```python
from build123d import *

# Parameters (mm, degrees)
SKETCH_W            = 110
SKETCH_H            = 110
PAD_DEPTH           = 1.5
PAD001_DEPTH        = 1
SKETCH002_R         = 6
SKETCH002_R_2       = 1.5
SKETCH002_R_3       = 5
SKETCH002_W         = 12
SKETCH002_H         = 7
SKETCH002_W_2       = 10
SKETCH002_H_2       = 1
PAD002_DEPTH        = 1
LINEARPATTERN_COUNT = 4
LINEARPATTERN_PITCH = 26.67


with BuildPart() as part:
    # Sketch → Pad (new body)
    with BuildSketch(Plane.XY):
        Rectangle(SKETCH_W, SKETCH_H)
    extrude(amount=PAD_DEPTH)

    # Sketch001 → Pad001 (join)
    with BuildSketch(Plane(origin=(0, 0, 0), x_dir=(1, 0, 0), z_dir=(0, 0, -1))):
        with BuildLine():
            Line((-49.8, 53.8), (49.8, 53.8))
            ThreePointArc((53.8, 49.8), (52.628427, 52.628427), (49.8, 53.8))
            Line((53.8, 49.8), (53.8, -49.8))
            ThreePointArc((49.8, -53.8), (52.628427, -52.628427), (53.8, -49.8))
            Line((49.8, -53.8), (-49.8, -53.8))
            ThreePointArc((-53.8, -49.8), (-52.628427, -52.628427), (-49.8, -53.8))
            Line((-53.8, -49.8), (-53.8, 49.8))
            ThreePointArc((-49.8, 53.8), (-52.628427, 52.628427), (-53.8, 49.8))
        make_face()
        with BuildLine():
            Line((-49.8, 52.8), (49.8, 52.8))
            ThreePointArc((52.8, 49.8), (51.92132, 51.92132), (49.8, 52.8))
            Line((52.8, 49.8), (52.8, -49.8))
            ThreePointArc((49.8, -52.8), (51.92132, -51.92132), (52.8, -49.8))
            Line((49.8, -52.8), (-49.8, -52.8))
            ThreePointArc((-52.8, -49.8), (-51.92132, -51.92132), (-49.8, -52.8))
            Line((-52.8, -49.8), (-52.8, 49.8))
            ThreePointArc((-49.8, 52.8), (-51.92132, 51.92132), (-52.8, 49.8))
        make_face(mode=Mode.SUBTRACT)
    extrude(amount=PAD001_DEPTH)

    # Sketch002 → Pad002 (join)
    with BuildSketch(Plane(origin=(0, 0, 0), x_dir=(1, 0, 0), z_dir=(0, 0, -1))):
        with Locations((-40.005, 40.005)):
            Circle(SKETCH002_R)
        with BuildLine():
            ThreePointArc((-36.42415, 36.515371), (-43.218938, 43.835222), (-37.190194, 35.872583))
            Line((-37.190194, 35.872583), (-38.925721, 37.940903))
            ThreePointArc((-38.888744, 38.363553), (-38.994766, 38.159886), (-38.925721, 37.940903))
            Line((-38.888744, 38.363553), (-38.582326, 38.620668))
            ThreePointArc((-38.159676, 38.583691), (-38.363343, 38.689713), (-38.582326, 38.620668))
            Line((-36.42415, 36.515371), (-38.159676, 38.583691))
        make_face(mode=Mode.SUBTRACT)
        with Locations((-40.005, 49.505)):
            Circle(SKETCH002_R_2)
        with Locations((-40.005, 25)):
            Circle(SKETCH002_R_2)
        with Locations((-40.005, -30.505)):
            Circle(SKETCH002_R_2)
        with Locations((-40.005, -40.005)):
            Circle(SKETCH002_R_3)
        with BuildLine():
            ThreePointArc((-39.255, 18.1), (-40.005, 18.85), (-40.755, 18.1))
            Line((-40.755, 18.1), (-40.755, 4.5))
            Line((-40.755, 4.5), (-39.255, 4.5))
            Line((-39.255, 18.1), (-39.255, 4.5))
        make_face()
        with BuildLine():
            ThreePointArc((-40.755, -18.1), (-40.005, -18.85), (-39.255, -18.1))
            Line((-39.255, -4.5), (-39.255, -18.1))
            Line((-40.755, -4.5), (-39.255, -4.5))
            Line((-40.755, -18.1), (-40.755, -4.5))
        make_face()
        with Locations((-40.005, 0)):
            Rectangle(SKETCH002_W, SKETCH002_H)
        with Locations((-40.005, 0)):
            Rectangle(SKETCH002_W_2, SKETCH002_H_2, mode=Mode.SUBTRACT)
    pad002 = extrude(amount=PAD002_DEPTH)

    # LinearPattern: Pad002 ×4
    with Locations(*[(i * LINEARPATTERN_PITCH, 0, 0) for i in range(1, LINEARPATTERN_COUNT)]):
        add(pad002)


solid = part.part
```
Geometry check sheet. Reference: the model listing, model coordinates, mm. A direction names the side the tool comes from. Coordinates: 2 decimals unless noted, no trailing zeros. Order: outer loops, then holes, each group sorted by start corner. A loop starts at its lowest first (then second) coordinate and runs counter-clockwise, first axis right, second up. Notation, with made-up numbers: (-33, -5) - (-20, -5) arc R29 ccw to (-20, 24) - close; hole circle Ø9 at (-15, 12). An arc over 180 degrees is marked (long way). Answer in a Markdown table with one row per item. Add a question column.
1. Draft check along Y on faces 3 (the face through (-13, 30, -1)), 4 (the face through (40.697, 31.836, -0.493)). Enter one of: +Y half, -Y half, draft (parallel to the pull), parting line (faces both ways), or undercut.
2. Material ranges on L1, parallel to X at y = -14, z = -0.05 (3 decimals); L2, parallel to Z at x = 14.5, y = 25; L3, parallel to Y at x = -8, z = -0.1, recorded low to high. Write a range as [from, to].
3. Section check A-A (y = 24.5). Enter the section's corners in (x, z), plus the area to 3 significant figures.
4. Access from +Z, -Z, +X, -X, +Y, -Y to the whole of each face (thin tool, end or side, straight path). Record for faces 1 (the face through (-51.94, 51.9, -0.49)), 2 (the face through (-13, -25, -1)).
5. Gauge pin test, flat ends, axial feed: pin 1 Ø0.8 at (y, z) = (-0.5, -0.5) entering from +X; pin 2 Ø0.8 at (x, y) = (-15.5, 0) entering from -Z; pin 3 Ø0.5 at (y, z) = (13, -0.5) entering from -X. Record the tip position at first contact, or that the pin passes through.
6. Section check C-C (y = -25). Enter the section's corners in (x, z) (3 decimals), plus the area to 3 significant figures.
Data:
| question | item | result |
|---|---|---|
| 1 | face 3 | draft |
| 1 | face 4 | undercut |
| 2 | L1 | x = [-53.8, -52.8], [-40.755, -39.255], [-14.085, -12.585], [12.585, 14.085], [39.255, 40.755], [52.8, 53.8] |
| 2 | L2 | z = [0, 1.5] |
| 2 | L3 | y = [-53.8, -52.8], [-42.75, -37.26], [-3.5, 3.5], [52.8, 53.8] |
| 3 | outline | (-55, 0) - (-53.8, 0) - (-53.8, -1) - (-52.8, -1) - (-52.8, 0) - (52.8, 0) - (52.8, -1) - (53.8, -1) - (53.8, 0) - (55, 0) - (55, 1.5) - (-55, 1.5) - close |
| 3 | area | 167 mm² |
| 4 | face 1 | -Z |
| 4 | face 2 | -Z, +X, -X, +Y, -Y |
| 5 | pin 1 | stops at x = 53.8 |
| 5 | pin 2 | stops at z = 0 |
| 5 | pin 3 | stops at x = -53.8 |
| 6 | outline | (-55, 0) - (-53.8, 0) - (-53.8, -1) - (-52.8, -1) - (-52.8, 0) - (-41.505, 0) - (-41.505, -1) - (-38.505, -1) - (-38.505, 0) - (-14.835, 0) - (-14.835, -1) - (-11.835, -1) - (-11.835, 0) - (11.835, 0) - (11.835, -1) - (14.835, -1) - (14.835, 0) - (38.505, 0) - (38.505, -1) - (41.505, -1) - (41.505, 0) - (52.8, 0) - (52.8, -1) - (53.8, -1) - (53.8, 0) - (55, 0) - (55, 1.5) - (-55, 1.5) - close |
| 6 | area | 179 mm² |
